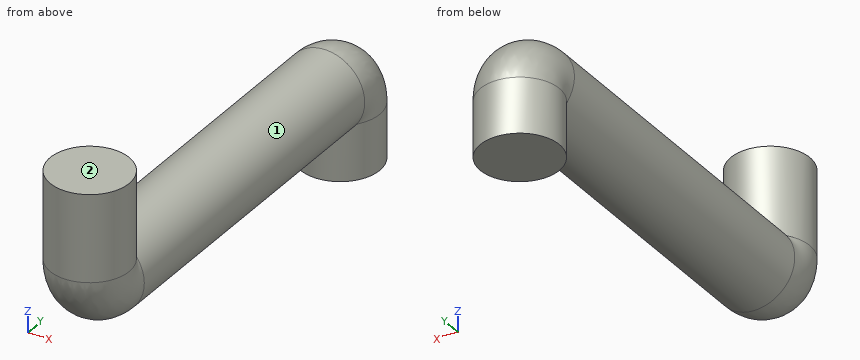
Autodesk Inventor part; units mm, degrees
ref_plane "YZ Plane" through (0, 0, 0) normal (1, 0, 0) x (0, 1, 0)
ref_plane "XZ Plane" through (0, 0, 0) normal (0, 1, 0) x (-1, 0, 0)
ref_plane "XY Plane" through (0, 0, 0) normal (0, 0, 1) x (1, 0, 0)
ref_plane "Work Plane1" through (-527.9617, -1874.6232, 239.2901) normal (0, 0, 1) x (1, 0, 0)
sketch "Sketch7" plane through (-527.9617, -1874.6232, 239.2901) normal (0, 0, 1) x (1, 0, 0)
  circle A0 centre (0, 0) radius 25
  point P0 (527.9617, 1874.6232)
  dimension "d25" = 50
sketch3d "3D Sketch6"
  line L0 (-527.9617, -1874.6232, 239.2901) -> (-527.9617, -1874.6232, 274.2901)
  arc A0 (-527.9617, -1874.6232, 274.2901) -> (-527.9617, -1889.6232, 289.2901) centre (-527.9617, -1889.6232, 274.2901) ccw
  line L1 (-527.9617, -1889.6232, 289.2901) -> (-527.9617, -2109.6232, 289.2901)
  arc A1 (-527.9617, -2109.6232, 289.2901) -> (-527.9617, -2124.6232, 304.2901) centre (-527.9617, -2109.6232, 304.2901) ccw
  line L2 (-527.9617, -2124.6232, 304.2901) -> (-527.9617, -2124.6232, 359.2901)
  dimension "d22" = 50
  dimension "d23" = 250
  dimension "d24" = 70
  dimension "d26" = 15
  dimension "d27" = 15
sweep "Sweep1" add profiles "Sketch7" path "3D Sketch6"
properties part number "Exhaust"
CAD build for the part. Positions are in the model's coordinates, mm. Face numbers are marked on the shaded views. A direction names the side the tool comes from. Coordinates: 2 decimals unless noted, no trailing zeros. Order: outer loops, then holes, each group sorted by start corner. A loop starts at its lowest first (then second) coordinate and runs counter-clockwise, first axis right, second up. Notation, with made-up numbers: (20, 24) - (40, 24) arc R13 cw to (40, 35) - close; hole circle Ø8 at (27.25, 50). An arc over 180 degrees is marked (long way). Answer in a Markdown table with one row per item.
1. Flat gauge pins, fed straight in: P1, Ø2, axis at x = -542, y = -1897, coming from the +Z side; P2, Ø10, axis at y = -1989.5, z = 270.5, coming from the -X side; P3, Ø6, axis at x = -539.5, z = 320, coming from the +Y side. Where does each tip first touch, or does it go through?
Answer:
| item | result |
|---|---|
| P1 | z = 310.62 |
| P2 | x = -548.81 |
| P3 | y = -2101.13 |
2. Slice it at B-B, the plane z = 335. List the corners of the cut face in (x, y), then the cut area to 3 significant figures.
Answer:
| item | result |
|---|---|
| outline | circle Ø50 at (-527.96, -2124.62) |
| area | 1,960 mm² |
3. Slice it at C-C, the plane y = -1941. List the corners of the cut face in (x, z), then the cut area to 3 significant figures.
Answer:
| item | result |
|---|---|
| outline | circle Ø50 at (-527.96, 289.29) |
| area | 1,960 mm² |
4. Drill centre lines: L1, parallel to X at y = -1933.5, z = 291; L2, parallel to Z at x = -537.5, y = -2078.5; L3, parallel to Y at x = -511.5, z = 297.5. Where is each one in solid material? Low to high. Write a range as from..to.
Answer:
| item | result |
|---|---|
| L1 | -552.9..-503.02 |
| L2 | 266.18..312.4 |
| L3 | -2142.75..-1865.03 |
5. 3-axis set-ups, long thin cutter, end or side, ignore diameter. For the marked faces 1 and 2: which of +Z, -Z, +X, -X, +Y, -Y reach the whole face in a straight line?
Answer:
| item | result |
|---|---|
| face 1 | none |
| face 2 | +Z, +X, -X, +Y, -Y |
